```python
from build123d import *

# Parameters (mm, degrees)
F3_DEPTH = 25.4
F5_D     = 9.525


# Not quite as in the source:
# - a length typed as a fraction of an inch, garbled in the dataset ("3 / 203.2 mm" for 3/8 in), is restored


with BuildPart() as f1:
    # F0 (on Front) → F1 (revolve)
    with BuildSketch(Plane.XZ):
        Polygon((0, -114.3), (0, 0), (-25.4, 0), (-25.4, -12.7), (-38.1, -12.7), (-38.1, -10.16), (-76.2, -10.16), (-76.2, -22.86), (-28.575, -22.86), (-28.575, -25.4), (-12.7, -25.4), (-12.7, -101.6), (-9.525, -101.6), (-9.525, -114.3), align=None)
    revolve(axis=Axis((0, 0, -53.3123221248), (0, 0, -1)))

    # F2 (on face) → F3 (cut)
    with BuildSketch(Plane.XY.offset(-10.16)):
        with BuildLine():
            ThreePointArc((-33.332184286, -18.4546875), (0, -38.1), (33.332184286, -18.4546875))
            ThreePointArc((33.332184286, -18.4546875), (0, -9.525), (-33.332184286, -18.4546875))
        make_face()
    extrude(amount=F3_DEPTH, mode=Mode.SUBTRACT)

    # F5 (through all)
    with Locations(Plane.XY.offset(-10.16)):
        with Locations((0, -57.15)):
            Hole(F5_D / 2)


solid = f1.part
```
Verification items for the finished model (mm, model axes). A direction names the side the tool comes from. Round coordinates to 2 decimals unless told otherwise and drop trailing zeros. Order: outer loops, then holes, each group sorted by start corner. A loop starts at its lowest first (then second) coordinate and runs counter-clockwise, first axis right, second up.
1) Cross-section at D-D, the plane x = 17. Record the cut outline in (y, z).
Geometry says:
outline: (-74.28, -22.86) - (-22.97, -22.86) - (-22.97, -25.4) - (22.97, -25.4) - (22.97, -22.86) - (74.28, -22.86) - (74.28, -10.16) - (34.1, -10.16) - (34.1, -12.7) - (18.87, -12.7) - (18.87, 0) - (-11.73, 0) - (-11.73, -10.16) - (-18.87, -10.16) - (-18.87, -12.7) - (-34.1, -12.7) - (-34.1, -10.16) - (-74.28, -10.16) - close
2) Draft check along X on faces 1 (the flat face through (16, 35, -10.16)), 2 (the cylindrical face through (2.75, -12.4, -64.03)), 3 (the cylindrical face through (30.235, -23.183, -11.412)), 4 (the flat face through (25, -8, -12.7)). Enter one of: +X half, -X half, draft (parallel to the pull), parting line (faces both ways), or undercut.
Geometry says:
face 1: draft
face 2: parting line
face 3: undercut
face 4: undercut
3) Tool access check on faces 5 (the cylindrical face through (0.31, -9.526, -5.151)), 6 (the flat face through (-5, 9, -101.6)), 7 (the cylindrical face through (60.47, -46.367, -16.599)), 8 (the cylindrical face through (-13.65, 21.42, -6.44)). Record the directions out of +Z, -Z, +X, -X, +Y, -Y that give a thin tool (end or side, any length) a straight path to the whole face; none if there is none.
Geometry says:
face 5: +Z, -Y
face 6: -Z
face 7: +Z, -Z
face 8: +Z
4) Depth check by flat-ended pin: pin 1 (8.5 mm diameter, centred on x = 0, y = -57.15, fed in from +Z); pin 2 (5 mm diameter, centred on x = 7.5, y = -18.5, fed in from +Z); pin 3 (12 mm diameter, centred on y = 0, z = -67, fed in from -X); pin 4 (17 mm diameter, centred on x = 11.5, y = 7, fed in from -Z). Enter the tip coordinate at first touch or a pass-through.
Geometry says:
pin 1: passes through
pin 2: stops at z = -10.16
pin 3: stops at x = -12.7
pin 4: stops at z = -114.3
5) Cross-section at B-B, the plane y = 0. Record the cut outline in (x, z) (3 decimals).
Geometry says:
outline: (-76.2, -22.86) - (-28.575, -22.86) - (-28.575, -25.4) - (-12.7, -25.4) - (-12.7, -101.6) - (-9.525, -101.6) - (-9.525, -114.3) - (9.525, -114.3) - (9.525, -101.6) - (12.7, -101.6) - (12.7, -25.4) - (28.575, -25.4) - (28.575, -22.86) - (76.2, -22.86) - (76.2, -10.16) - (38.1, -10.16) - (38.1, -12.7) - (25.4, -12.7) - (25.4, 0) - (-25.4, 0) - (-25.4, -12.7) - (-38.1, -12.7) - (-38.1, -10.16) - (-76.2, -10.16) - close
6) Material ranges on line 1 (Y direction, x = 0, z = -11.35); line 2 (Y direction, x = 0, z = -15); line 3 (Z direction, x = -49.5, y = 42), recorded low to high.
Geometry says:
line 1: y = -76.2 to -61.91, -52.39 to -38.1, -25.4 to 25.4, 38.1 to 76.2
line 2: y = -76.2 to -61.91, -52.39 to 76.2
line 3: z = -22.86 to -10.16
7) Cross-section at C-C, the plane y = -57.15. Record the cut outline in (x, z).
Geometry says:
outline: (-50.4, -22.86) - (-4.76, -22.86) - (-4.76, -10.16) - (-50.4, -10.16) - close; (4.76, -22.86) - (50.4, -22.86) - (50.4, -10.16) - (4.76, -10.16) - close
